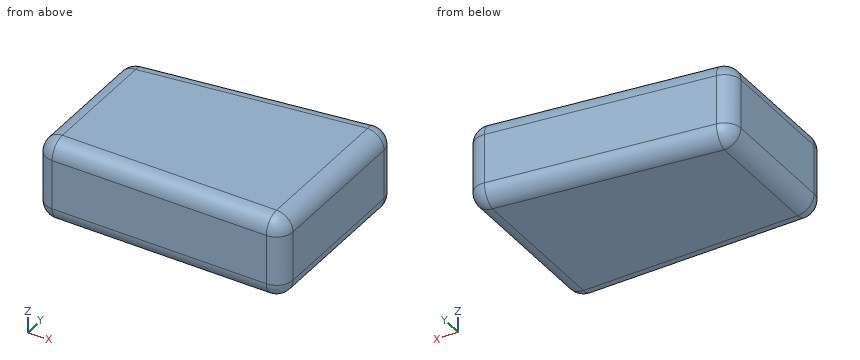
```python
from build123d import *

# Parameters (mm, degrees)
EXTRUDE_DEPTH = 5
FILLET_R      = 1


with BuildPart() as part:
    # Sketch → Extrude (new body)
    with BuildSketch(Plane.XY):
        Polygon((-7.5, 4.5), (-7.5, -4.5), (7.5, -4.5), (7.5, 6.5), align=None)
    extrude(amount=EXTRUDE_DEPTH)

    # Fillet
    fillet_edges = [part.edges().sort_by_distance(p)[0] for p in [
        (-7.5, 4.5, 2.5),
        (-7.5, -4.5, 2.5),
        (-7.5, 0, 0),
        (-7.5, 0, 5),
        (7.5, -4.5, 2.5),
        (0, -4.5, 0),
        (0, -4.5, 5),
        (7.5, 6.5, 2.5),
        (7.5, 1, 0),
        (7.5, 1, 5),
        (0, 5.5, 0),
        (0, 5.5, 5),
    ]]
    fillet(fillet_edges, radius=FILLET_R)


solid = part.part
```
Could you check a few things on this model? Use its own coordinates, in mm. Coordinates: 2 decimals unless noted, no trailing zeros. Loops run counter-clockwise (first coordinate to the right, second up) from the corner with the lowest first, then second, coordinate; pieces in that order, holes last.
1) Imagine slicing it at A-A (z = 2.95). List the corners of the cut face in (x, y) for me.
Reported:
outline: (-7.5, -3.5) arc R1 ccw to (-6.5, -4.5) - (6.5, -4.5) arc R1 ccw to (7.5, -3.5) - (7.5, 5.36) arc R1 ccw to (6.37, 6.35) - (-6.63, 4.62) arc R1 ccw to (-7.5, 3.62) - close
2) Will this pin go through, and if not, where does the flat tip stop? pin 1 Ø3 at (x, y) = (5.5, 1) entering from -Z.
Reported:
pin 1: stops at z = 0
3) Imagine slicing it at B-B (z = 0.7). List the corners of the cut face in (x, y) for me, and give its area (3 significant figures).
Reported:
outline: (-7.45, -3.5) arc R0.95 ccw to (-6.5, -4.45) - (6.5, -4.45) arc R0.95 ccw to (7.45, -3.5) - (7.45, 5.36) arc R0.95 ccw to (6.37, 6.3) - (-6.63, 4.57) arc R0.95 ccw to (-7.45, 3.62) - close
area: 147 mm2
4) Please list where these lines run through material, in increasing order: line 1 along Y through (x, z) = (-3.75, 2.95); line 2 along Y through (x, z) = (-1.25, 2.85); line 3 along X through (y, z) = (-2, 4.65).
Reported:
line 1: y = -4.5 to 5
line 2: y = -4.5 to 5.33
line 3: x = -7.26 to 7.26
